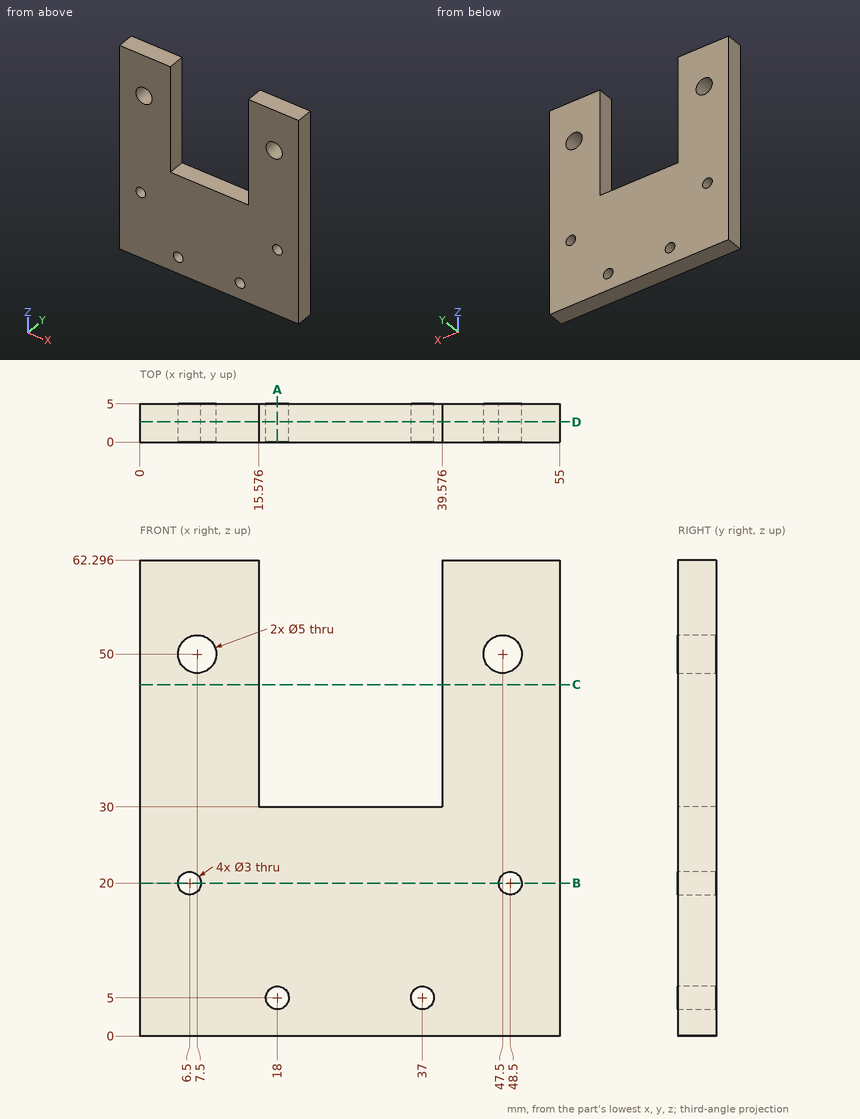
Check sheet for the drawn part. Datum: minimum x, y, z corner. Units: mm. Round coordinates to 2 decimals unless told otherwise and drop trailing zeros. Write each loop counter-clockwise with the first axis right and the second up, starting at its lowest first coordinate (ties: lowest second). Pieces come first, ordered by that corner, then holes. Notation, with made-up numbers: (-28.5, -19) -> (-0.5, -19) arc R24 ccw to (-0.5, 0) -> close; hole circle Ø11 at (-35.75, 38). An arc over 180 degrees is marked (long way). One line per item, written item: value. Start each with the question number.
(1) Scan lines: line 1 (X direction, y = 3.45, z = 20); line 2 (X direction, y = 2.4, z = 50); line 3 (X direction, y = 4.15, z = 45). Record each from-to range of solid material in increasing order. Write a range as [from, to].
(2) Cross-section at D-D, the plane y = 2.65. Record the cut outline in (x, z), and give its area (3 significant figures).
(3) Cross-section at A-A, the plane x = 18. Record the cut outline in (y, z).
(4) Cross-section at B-B, the plane z = 20. Record the cut outline in (x, y).
(5) Cross-section at C-C, the plane z = 46. Record the cut outline in (x, y).
(6) Go/stop test with a flat-tipped pin: pin 1 Ø2.5 at (x, y) = (23, 2.5) entering from +Z. Record where the tip stops, or that it passes through.
Answer:
1. line 1: [0, 5], [8, 47], [50, 55]
1. line 2: [0, 5], [10, 15.58], [39.58, 45], [50, 55]
1. line 3: [0, 15.58], [39.58, 55]
2. outline: (0, 0) -> (55, 0) -> (55, 62.3) -> (39.58, 62.3) -> (39.58, 30) -> (15.58, 30) -> (15.58, 62.3) -> (0, 62.3) -> close; hole circle Ø3 at (6.5, 20); hole circle Ø5 at (7.5, 50); hole circle Ø3 at (18, 5); hole circle Ø3 at (37, 5); hole circle Ø5 at (47.5, 50); hole circle Ø3 at (48.5, 20)
2. area: 2,580 mm²
3. outline: (0, 0) -> (5, 0) -> (5, 3.5) -> (0, 3.5) -> close; (0, 6.5) -> (5, 6.5) -> (5, 30) -> (0, 30) -> close
4. outline: (0, 0) -> (5, 0) -> (5, 5) -> (0, 5) -> close; (8, 0) -> (47, 0) -> (47, 5) -> (8, 5) -> close; (50, 0) -> (55, 0) -> (55, 5) -> (50, 5) -> close
5. outline: (0, 0) -> (15.58, 0) -> (15.58, 5) -> (0, 5) -> close; (39.58, 0) -> (55, 0) -> (55, 5) -> (39.58, 5) -> close
6. pin 1: z = 30
